For this review, take the finished solid that the model builds, in its own axes (mm). A direction names the side the tool comes from. Round coordinates to 2 decimals unless told otherwise and drop trailing zeros. Loops run counter-clockwise (first coordinate to the right, second up) from the corner with the lowest first, then second, coordinate; pieces in that order, holes last.
1. To check wall thickness, follow line 1 along X through (y, z) = (-13, 6); line 2 along X through (y, z) = (7.5, 4.5); line 3 along Y through (x, z) = (8, -3.4). State the ranges of each line that lie inside material, in increasing order.
2. Tool access review of faces 5 (the flat face through (-8, -7, 5)), 6 (the flat face through (-4, 2, 5)), 7 (the cylindrical face through (-7.45, -9.43, 4.4)), 8 (the flat face through (0, 10, 0)), 9 (the cylindrical face through (12.972, -11.906, 9.195)): name each direction out of +Z, -Z, +X, -X, +Y, -Y from which nothing blocks a thin tool from reaching the whole face with its end or side.
3. Clearance check with flat-ended pins moving along their axes: pin 1 Ø5 at (x, z) = (0, 9.5) entering from +Y; pin 2 Ø1.3 at (x, y) = (-6.5, -6) entering from +Z; pin 3 Ø3 at (x, y) = (8, 5.28) entering from -Z; pin 4 Ø1 at (x, z) = (2, 3.5) entering from -Y. State where each tip first meets the part, or that it passes through.
4. Consider section C-C on z = -3. State the section outline as (x, y) points.
5. Draft analysis for pull direction X (two halves, no side actions). For faces 1 (the flat face through (-11, -11.6, 6.5)), 2 (the flat face through (15, -3, 2)), 3 (the cylindrical face through (-14, 8, 0)), 4 (the cylindrical face through (-0.056, -10.975, 3.921)), state which applies: released by +X, released by -X, zero draft, split by the parting line, or undercut.
6. Consider section A-A on x = 0. State the section outline as (y, z) points.
7. Consider section D-D on x = -13. State the section outline as (y, z) points, then the cut area to 3 significant figures.
8. Consider section B-B on x = -8. State the section outline as (y, z) points, then the cut area to 3 significant figures.
from build123d import *

# Parameters (mm, degrees)
F0_W      = 30
F0_H      = 20
F0_R      = 1.6
F1_DEPTH  = 5
F3_DEPTH  = 30
F7_DEPTH  = 7
F9_DEPTH  = 7
F10_SIZE  = 2.5
F11_R     = 5
F12_R     = 1.6200998357
F13_DEPTH = 30.001
F14_R     = 2
F15_DEPTH = 4.3


with BuildPart() as f1:
    # F0 (on Top) → F1 (new body)
    with BuildSketch(Plane.XY):
        Rectangle(F0_W, F0_H)
        with Locations((-8, 5.2767994255)):
            Circle(F0_R, mode=Mode.SUBTRACT)
        with Locations((0, 0.0767994255)):
            Circle(F0_R, mode=Mode.SUBTRACT)
        with Locations((8, 5.2767994255)):
            Circle(F0_R, mode=Mode.SUBTRACT)
    extrude(amount=F1_DEPTH)

    # F2 (on face) → F3 (join, through all)
    with BuildSketch(Plane(origin=(-15, 0, 0), x_dir=(0, -1, 0), z_dir=(-1, 0, 0))):
        with BuildLine():
            ThreePointArc((13.1, 5), (15.2920310217, 5.9079689783), (16.2, 8.1))
            ThreePointArc((16.2, 8.1), (13.1, 11.2), (10, 8.1))
            ThreePointArc((10, 8.1), (10.9079689783, 5.9079689783), (13.1, 5))
        make_face()
        with BuildLine():
            ThreePointArc((13.1, 5), (10.9079689783, 5.9079689783), (10, 8.1))
            ThreePointArc((10, 8.1), (8.1808280522, 5.8625059643), (5.4291286506, 5))
            Line((5.4291286506, 5), (10, 5))
            Line((10, 5), (10, 1.816622098))
            ThreePointArc((10, 1.816622098), (10.998268655, 3.9455916428), (13.1, 5))
        make_face()
    extrude(amount=-F3_DEPTH)

    # F6 (on offset) → F7 (cut)
    with BuildSketch(Plane.YZ.offset(11)):
        with BuildLine():
            ThreePointArc((-13.1, 5), (-10.9079689783, 5.9079689783), (-10, 8.1))
            ThreePointArc((-10, 8.1), (-15.2920310217, 10.2920310217), (-13.1, 5))
        make_face()
        with BuildLine():
            ThreePointArc((-5.4291286506, 5), (-8.1808280522, 5.8625059643), (-10, 8.1))
            ThreePointArc((-10, 8.1), (-10.9079689783, 5.9079689783), (-13.1, 5))
            ThreePointArc((-13.1, 5), (-10.998268655, 3.9455916428), (-10, 1.816622098))
            Line((-10, 1.816622098), (-10, 5))
            Line((-10, 5), (-5.4291286506, 5))
        make_face()
        with BuildLine():
            Line((-5.3136004135, 5), (-5.4291286506, 5))
            ThreePointArc((-5.4291286506, 5), (-5.371364532, 4.9996666743), (-5.3136004135, 5))
        make_face()
    extrude(amount=-F7_DEPTH, mode=Mode.SUBTRACT)

    # F8 (on offset) → F9 (cut)
    with BuildSketch(Plane(origin=(-11, 0, 0), x_dir=(0, -1, 0), z_dir=(-1, 0, 0))):
        with BuildLine():
            ThreePointArc((13.1, 5), (15.2920310217, 5.9079689783), (16.2, 8.1))
            ThreePointArc((16.2, 8.1), (13.1, 11.2), (10, 8.1))
            ThreePointArc((10, 8.1), (10.9079689783, 5.9079689783), (13.1, 5))
        make_face()
        with BuildLine():
            ThreePointArc((5.3136004135, 5), (5.371364532, 4.9996666743), (5.4291286506, 5))
            Line((5.4291286506, 5), (5.3136004135, 5))
        make_face()
        with BuildLine():
            ThreePointArc((13.1, 5), (10.9079689783, 5.9079689783), (10, 8.1))
            ThreePointArc((10, 8.1), (8.1808280522, 5.8625059643), (5.4291286506, 5))
            Line((5.4291286506, 5), (10, 5))
            Line((10, 5), (10, 1.816622098))
            ThreePointArc((10, 1.816622098), (10.998268655, 3.9455916428), (13.1, 5))
        make_face()
    extrude(amount=-F9_DEPTH, mode=Mode.SUBTRACT)

    # F10
    f10_edges = [f1.edges().sort_by_distance(p)[0] for p in [
        (-9.6, 5.276799, 5),
        (-1.6, 0.076799, 5),
        (6.4, 5.276799, 5),
    ]]
    chamfer(f10_edges, length=F10_SIZE)

    # F11
    f11_edges = [f1.edges().sort_by_distance(p)[0] for p in [
        (-15, 10, 2.5),
        (15, 10, 2.5),
    ]]
    fillet(f11_edges, radius=F11_R)

    # F12 (on face) → F13 (cut, through all)
    with BuildSketch(Plane(origin=(-15, 0, 0), x_dir=(0, -1, 0), z_dir=(-1, 0, 0))):
        with Locations((13.1, 8.1)):
            Circle(F12_R)
    extrude(amount=-F13_DEPTH, mode=Mode.SUBTRACT)

    # F14
    f14_edges = [f1.edges().sort_by_distance(p)[0] for p in [
        (-7.5, -10, 5),
        (7.5, -10, 5),
    ]]
    fillet(f14_edges, radius=F14_R)

    # F15 (add): a face of the model
    f15_faces = [f1.faces().sort_by_distance(p)[0] for p in [
        (14.6394448725, -2.5, 0),
    ]]
    extrude(f15_faces, amount=F15_DEPTH)


solid = f1.part
Resolved:
1. line 1: x = -15 to -11, -4 to 4, 11 to 15
1. line 2: x = -14.33 to -10.83, -5.17 to 5.17, 10.83 to 14.33
1. line 3: y = -10 to 3.68, 6.88 to 10
2. face 5: +Z, +Y, -Y
2. face 6: +Z, +X, -X, +Y
2. face 7: +Z, -Y
2. face 8: +Z, -Z, +X, -X, +Y
2. face 9: +X, -X
3. pin 1: stops at y = -9.37
3. pin 2: stops at z = 5
3. pin 3: passes through
3. pin 4: stops at y = -11.05
4. outline: (-15, -10) - (15, -10) - (15, 5) arc R5 ccw to (10, 10) - (-10, 10) arc R5 ccw to (-15, 5) - close; hole circle Ø3.2 at (-8, 5.28); hole circle Ø3.2 at (0, 0.08); hole circle Ø3.2 at (8, 5.28)
5. face 1: undercut
5. face 2: released by +X
5. face 3: released by -X
5. face 4: zero draft
6. outline: (-13.1, 5) arc R3.59 cw to (-10, 1.82) - (-10, -4.3) - (-1.52, -4.3) - (-1.52, 2.5) - (-4.02, 5) - (-5.43, 5) arc R5.01 cw to (-10, 8.1) arc R3.1 ccw (long way) to start; (1.68, -4.3) - (10, -4.3) - (10, 5) - (4.18, 5) - (1.68, 2.5) - close; hole circle Ø3.24 at (-13.1, 8.1)
7. outline: (-13.1, 5) arc R3.59 cw to (-10, 1.82) - (-10, -4.3) - (9, -4.3) - (9, 5) - (-5.43, 5) arc R5.01 cw to (-10, 8.1) arc R3.1 ccw (long way) to start; hole circle Ø3.24 at (-13.1, 8.1)
7. area: 207 mm2
8. outline: (-10, -4.3) - (3.68, -4.3) - (3.68, 2.5) - (1.18, 5) - (-5.31, 5) arc R5.01 cw to (-5.43, 5) - (-8, 5) arc R2 ccw to (-10, 3) - close; (6.88, -4.3) - (10, -4.3) - (10, 5) - (9.38, 5) - (6.88, 2.5) - close
8. area: 149 mm2
